Can you work these out from the model? Positions are in its coordinate system, mm. A direction names the side the tool comes from. Coordinates: 2 decimals unless noted, no trailing zeros. Order: outer loops, then holes, each group sorted by start corner. A loop starts at its lowest first (then second) coordinate and runs counter-clockwise, first axis right, second up. Notation, with made-up numbers: (-14.5, 16) -> (39.5, 16) arc R25 ccw to (39.5, 39) -> close; hole circle Ø10 at (-37.75, 42.25). An arc over 180 degrees is marked (long way). Use a Markdown table: item, result. Add a question column.
1. Suppose I cut it at C-C, the plane x = 63. List the corners of the cut face in (y, z) for me.
2. For faces 1 (the flat face through (131.762, 6, -171)), 2 (the flat face through (190.5, 6, -142)), 3 (the flat face through (151, 6, -190.5)), 4 (the flat face through (169.862, 6, -172)), 5 (the flat face through (76.2, 6, -28)), which set-ups out of +Z, -Z, +X, -X, +Y, -Y let a thin tool reach every point of the face, with its end or its side?
3. If I drill on line 1 along X through (y, z) = (2, -177.5); line 2 along X through (y, z) = (7.25, -27.5); line 3 along Z through (x, y) = (150, 5), over which ranges is the centre line in solid material (lowest first)? Write a range as from..to.
4. Suppose I cut it at A-A, the plane y = 5.5. List the corners of the cut face in (x, z) for me, then the cut area to 3 significant figures.
5. Suppose I cut it at B-B, the plane z = -20.5. List the corners of the cut face in (x, y) for me.
6. For pin 1 Ø3.5 at (x, y) = (173.5, 7.5) entering from +Z; pin 2 Ø5 at (x, y) = (56.5, 8.5) entering from -Z; pin 3 Ø5 at (x, y) = (133, 4.5) entering from +Z, each with a flat end and sliding along its axis, tell me the tip position at first contact or that it passes through.
```python
from build123d import *

# Parameters (mm, degrees)
BOSS_EXTRUDE1_DEPTH = 11.557
FILLET1_R           = 5.08


with BuildPart() as part:
    # Sketch1 → Boss-Extrude1 (new body)
    with BuildSketch(Plane(origin=(0, 0, 0), x_dir=(1, 0, 0), z_dir=(0, 1, 0))):
        with BuildLine():
            Line((50.8, 25.4), (50.8, 152.4))
            Line((50.8, 152.4), (131.7625, 152.4))
            Line((131.7625, 152.4), (131.7625, 190.5))
            Line((131.7625, 190.5), (169.8625, 190.5))
            Line((169.8625, 190.5), (169.8625, 152.4))
            Line((169.8625, 152.4), (190.5, 152.4))
            Line((190.5, 152.4), (190.5, 127))
            Line((190.5, 127), (152.4, 127))
            ThreePointArc((152.4, 127), (98.518463274, 104.681536726), (76.2, 50.8))
            Line((76.2, 50.8), (76.2, 0))
            Line((76.2, 0), (0, 0))
            Line((0, 0), (0, 25.4))
            Line((0, 25.4), (50.8, 25.4))
        make_face()
    extrude(amount=BOSS_EXTRUDE1_DEPTH)

    # Fillet1
    fillet1_edges = [part.edges().sort_by_distance(p)[0] for p in [
        (190.5, 5.7785, -127),
        (76.2, 5.7785, 0),
        (0, 5.7785, 0),
    ]]
    fillet(fillet1_edges, radius=FILLET1_R)


solid = part.part
```
Worked out:
| question | item | result |
|---|---|---|
| 1 | outline | (0, -152.4) -> (11.56, -152.4) -> (11.56, 0) -> (0, 0) -> close |
| 2 | face 1 | -Z, -X, +Y, -Y |
| 2 | face 2 | +Z, -Z, +X, +Y, -Y |
| 2 | face 3 | -Z, +X, -X, +Y, -Y |
| 2 | face 4 | -Z, +X, +Y, -Y |
| 2 | face 5 | +Z, +X, +Y, -Y |
| 3 | line 1 | x = 131.76..169.86 |
| 3 | line 2 | x = 50.8..76.2 |
| 3 | line 3 | z = -190.5..-126.96 |
| 4 | outline | (0, -25.4) -> (50.8, -25.4) -> (50.8, -152.4) -> (131.76, -152.4) -> (131.76, -190.5) -> (169.86, -190.5) -> (169.86, -152.4) -> (190.5, -152.4) -> (190.5, -132.08) arc R5.08 ccw to (185.42, -127) -> (152.4, -127) arc R76.2 cw to (76.2, -50.8) -> (76.2, -5.08) arc R5.08 ccw to (71.12, 0) -> (5.08, 0) arc R5.08 ccw to (0, -5.08) -> close |
| 4 | area | 10,700 mm² |
| 5 | outline | (0, 0) -> (76.2, 0) -> (76.2, 11.56) -> (0, 11.56) -> close |
| 6 | pin 1 | stops at z = -127 |
| 6 | pin 2 | stops at z = -152.4 |
| 6 | pin 3 | stops at z = -123.79 |
